Source: CAD feature listing. Evaluate the final solid. Frame: model axes, mm. Face numbers are marked on the shaded views. A direction names the side the tool comes from. Round coordinates to 2 decimals unless told otherwise and drop trailing zeros. Order: outer loops, then holes, each group sorted by start corner. A loop starts at its lowest first (then second) coordinate and runs counter-clockwise, first axis right, second up.
```python
from build123d import *

# Parameters (mm, degrees)
SKETCH1_R           = 63.5
BOSS_EXTRUDE1_DEPTH = 22.352
SKETCH2_R           = 19.05
CUT_EXTRUDE2_DEPTH  = 93.542487021
SKETCH3_R           = 4.3688
CUT_EXTRUDE4_DEPTH  = 93.542487021
SKETCH4_R           = 6.7437
CUT_EXTRUDE5_DEPTH  = 9.652
CHAMFER1_SIZE       = 1.524


with BuildPart() as part:
    # Sketch1 → Boss-Extrude1 (new body)
    with BuildSketch(Plane.YZ):
        with Locations(Location((0, 0, 0), (0, 0, 270))):
            Circle(SKETCH1_R)
    extrude(amount=BOSS_EXTRUDE1_DEPTH)

    # Sketch2 → Cut-Extrude2 (cut, through all)
    with BuildSketch(Plane.YZ):
        with Locations(Location((0, 0, 0), (0, 0, 270))):
            Circle(SKETCH2_R)
    extrude(amount=CUT_EXTRUDE2_DEPTH, mode=Mode.SUBTRACT)

    # Sketch3 → Cut-Extrude4 (cut, through all)
    with BuildSketch(Plane.YZ):
        with Locations(Location((53.975, 0, 0), (0, 0, 270))):
            Circle(SKETCH3_R)
        with Locations(Location((0, 53.975, 0), (0, 0, 270))):
            Circle(SKETCH3_R)
        with Locations(Location((-53.975, 0, 0), (0, 0, 270))):
            Circle(SKETCH3_R)
        with Locations(Location((0, -53.975, 0), (0, 0, 270))):
            Circle(SKETCH3_R)
    extrude(amount=CUT_EXTRUDE4_DEPTH, mode=Mode.SUBTRACT)

    # Sketch4 → Cut-Extrude5 (cut)
    with BuildSketch(Plane.YZ):
        with Locations(Location((53.975, 0, 0), (0, 0, 270))):
            Circle(SKETCH4_R)
        with Locations(Location((0, 53.975, 0), (0, 0, 270))):
            Circle(SKETCH4_R)
        with Locations(Location((-53.975, 0, 0), (0, 0, 270))):
            Circle(SKETCH4_R)
        with Locations(Location((0, -53.975, 0), (0, 0, 270))):
            Circle(SKETCH4_R)
    extrude(amount=CUT_EXTRUDE5_DEPTH, mode=Mode.SUBTRACT)

    # Chamfer1
    chamfer1_edges = [part.edges().sort_by_distance(p)[0] for p in [
        (0, 0, 63.5),
        (22.352, 0, 63.5),
    ]]
    chamfer(chamfer1_edges, length=CHAMFER1_SIZE)


solid = part.part
```
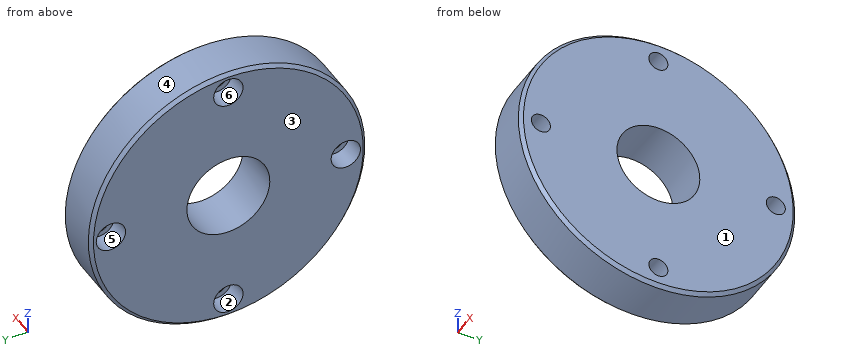
1. First-contact query: pin 1 (2 mm diameter, centred on x = 8.5, y = 49, fed in from -Z); pin 2 (8 mm diameter, centred on y = 0, z = 53.975, fed in from +X); pin 3 (11.5 mm diameter, centred on y = -53.975, z = 0, fed in from +X); pin 4 (11 mm diameter, centred on y = -53.975, z = 0, fed in from -X). Flat tips, straight axial feed; report the tip coordinate or a pass-through.
2. Line query: line 1 along Y through (x, z) = (3.75, 0); line 2 along Y through (x, z) = (11.75, 1); line 3 along Z through (x, y) = (2.75, -1.5). Output: solid intervals per line, ascending.
3. Section C-C on x = 13.25. Return loops of the section in (y, z) (3 decimals), plus the area to 3 significant figures.
4. Section A-A on y = 0. Return loops of the section in (x, z).
5. Access query for the marked faces 1 and 2. Directions: +Z, -Z, +X, -X, +Y, -Y. A direction counts if a zero-diameter tool reaches every point of the face in a straight line with its end or side. Return the directions, or none.
6. Pull-direction query (Z, two-part tool) for the marked faces 3, 4, 5 and 6; classes: released by +Z, released by -Z, zero draft, split by the parting line, or undercut.
7. Section D-D on x = 5.5. Return loops of the section in (y, z) (3 decimals), plus the area to 3 significant figures.
Result:
1. pin 1: stops at z = -41.57
1. pin 2: passes through
1. pin 3: stops at x = 22.35
1. pin 4: stops at x = 9.65
2. line 1: y = -63.5 to -60.72, -47.23 to -19.05, 19.05 to 47.23, 60.72 to 63.5
2. line 2: y = -63.49 to -58.23, -49.72 to -19.02, 19.02 to 49.72, 58.23 to 63.49
2. line 3: z = -63.48 to -60.55, -47.4 to -18.99, 18.99 to 47.4, 60.55 to 63.48
3. outline: circle Ø127 at (0, 0); hole circle Ø8.738 at (-53.975, 0); hole circle Ø38.1 at (0, 0); hole circle Ø8.738 at (0, -53.975); hole circle Ø8.738 at (0, 53.975); hole circle Ø8.738 at (53.975, 0)
3. area: 11,300 mm2
4. outline: (0, -61.98) - (1.52, -63.5) - (20.83, -63.5) - (22.35, -61.98) - (22.35, -58.34) - (9.65, -58.34) - (9.65, -60.72) - (0, -60.72) - close; (0, -47.23) - (9.65, -47.23) - (9.65, -49.61) - (22.35, -49.61) - (22.35, -19.05) - (0, -19.05) - close; (0, 19.05) - (22.35, 19.05) - (22.35, 49.61) - (9.65, 49.61) - (9.65, 47.23) - (0, 47.23) - close; (0, 60.72) - (9.65, 60.72) - (9.65, 58.34) - (22.35, 58.34) - (22.35, 61.98) - (20.83, 63.5) - (1.52, 63.5) - (0, 61.98) - close
5. face 1: +Z, -Z, +X, +Y, -Y
5. face 2: -X
6. face 3: zero draft
6. face 4: split by the parting line
6. face 5: undercut
6. face 6: undercut
7. outline: circle Ø127 at (0, 0); hole circle Ø13.487 at (-53.975, 0); hole circle Ø38.1 at (0, 0); hole circle Ø13.487 at (0, -53.975); hole circle Ø13.487 at (0, 53.975); hole circle Ø13.487 at (53.975, 0)
7. area: 11,000 mm2
